from build123d import *

# Parameters (mm, degrees)
SKETCH1_R           = 2.5
BOSS_EXTRUDE1_DEPTH = 2
THREAD1_PITCH       = 0.25


with BuildPart() as part:
    # Sketch1 → Boss-Extrude1 (new body)
    with BuildSketch(Plane(origin=(0, 0, 0), x_dir=(0, 0, -1), z_dir=(1, 0, 0))):
        Polygon((-2.651650429, 2.651650429), (0, 3.75), (2.651650429, 2.651650429), (3.75, 0), (2.651650429, -2.651650429), (0, -3.75), (-2.651650429, -2.651650429), (-3.75, 0), align=None)
        Circle(SKETCH1_R, mode=Mode.SUBTRACT)
    extrude(amount=BOSS_EXTRUDE1_DEPTH)

    # Thread1: the profile of Thread Profile1 profile screwed along a right-hand helix of 6 turns, 6 arcs to a turn; built about Z, then put on its axis
    thread1_z = Axis((0, 0, 0), (0, 0, 1))
    thread1_corners = [(2.4997, 0, -0.000173205), (2.635316469, 0, 0.078125), (2.635316469, 0, 0.109375), (2.4997, 0, 0.187673204)]
    with BuildLine(mode=Mode.PRIVATE) as thread1_profile:
        Line(thread1_corners[0], thread1_corners[1])
        Line(thread1_corners[1], thread1_corners[2])
        Line(thread1_corners[2], thread1_corners[3])
        Line(thread1_corners[3], thread1_corners[0])
    thread1_cap = Face(thread1_profile.wire())
    thread1_turn_angles = [0, 30, 60, 90, 120, 150, 180, 210, 240, 270, 300, 330, 360]
    thread1_turn_weights = [1, 0.8660254037844387, 1, 0.8660254037844387, 1, 0.8660254037844387, 1, 0.8660254037844387, 1, 0.8660254037844387, 1, 0.8660254037844387, 1]
    thread1_turn_rails = [Edge.make_bspline([Vector(p[0], p[1], 0).rotate(thread1_z, thread1_turn_angles[k]) / thread1_turn_weights[k] + Vector(0, 0, p[2] + THREAD1_PITCH * thread1_turn_angles[k] / 360) for k in range(13)], [0, 0, 0, 1, 1, 2, 2, 3, 3, 4, 4, 5, 5, 6, 6, 6], 2, thread1_turn_weights) for p in thread1_corners]
    thread1_turn_sides = [Face.make_surface_from_curves(thread1_turn_rails[p[0]], thread1_turn_rails[p[1]]) for p in [(0, 1), (1, 2), (2, 3), (3, 0)]]
    thread1 = Plane(origin=(2, 0, 0), x_dir=(0, 0, 1), z_dir=(-1, 0, 0)) * Solid(Shell([*[p.moved(Location((0, 0, THREAD1_PITCH * i))) for i in range(6) for p in thread1_turn_sides], thread1_cap, thread1_cap.rotate(thread1_z, 2160).moved(Location((0, 0, THREAD1_PITCH * 2160 / 360)))]))
    add(thread1, mode=Mode.SUBTRACT)


solid = part.part
Can you work these out from the model? Positions are in its coordinate system, mm. Round coordinates to 2 decimals unless told otherwise and drop trailing zeros. Loops run counter-clockwise (first coordinate to the right, second up) from the corner with the lowest first, then second, coordinate; pieces in that order, holes last. Notation, with made-up numbers: (-28, 65) - (2, 65) arc R16 cw to (2, 77) - close; hole circle Ø11 at (55.25, -9). An arc over 180 degrees is marked (long way). Write item = value, one per line. Start each with the question number.
(1) If we section it at B-B (z = -2.75): Please give me the cut outline in (x, y), and give its area (3 significant figures).
(2) For P1, Ø3, axis at y = 0, z = 0, coming from the +X side, with a flat end and sliding along its axis, tell me the tip position at first contact or that it passes through.
(3) If I drill on probe 1 along Z at (x, y) = (0.25, -2); probe 2 along Y at (x, z) = (0.25, 1); probe 3 along Z at (x, y) = (1.7, 3.5), over which ranges is the centre line in solid material (lowest first)? Write a range as [from, to].
(4) If we section it at A-A (y = 3): Please give me the cut outline in (x, z).
Ans:
q1.outline = (0, -2.41) - (2, -2.41) - (2, 2.41) - (0, 2.41) - close
q1.area = 9.66 mm²
q2.P1 = through
q3.probe_1 = [-2.92, -1.5], [1.5, 2.92]
q3.probe_2 = [-3.34, -2.29], [2.29, 3.34]
q3.probe_3 = [-0.6, 0.6]
q4.outline = (0, -1.81) - (2, -1.81) - (2, 1.81) - (0, 1.81) - close
